Can you work these out from the model? Positions are in its coordinate system, mm. Give positions to 0.01 mm unless a question says otherwise; leave off trailing zeros. Loops run counter-clockwise (first coordinate to the right, second up) from the corner with the lowest first, then second, coordinate; pieces in that order, holes last.
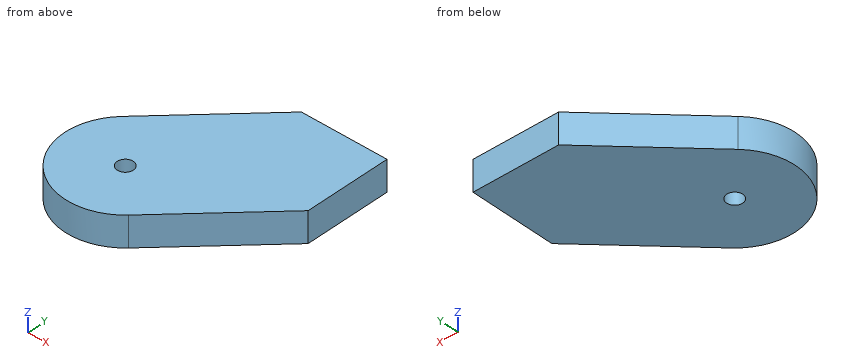
from build123d import *

# Parameters (mm, degrees)
F1_DEPTH = 25.4
F3_D     = 13.49248


with BuildPart() as f1:
    # F0 (on Top) → F1 (new body)
    with BuildSketch(Plane.XY):
        with BuildLine():
            Line((42.4579510314, 114.3), (-35.9210244843, 35.9210244843))
            ThreePointArc((-35.9210244843, 35.9210244843), (-35.9210244843, -35.9210244843), (35.9210244843, -35.9210244843))
            Line((35.9210244843, -35.9210244843), (114.3, 42.4579510314))
            Line((114.3, 42.4579510314), (114.3, 114.3))
            Line((114.3, 114.3), (42.4579510314, 114.3))
        make_face()
    extrude(amount=F1_DEPTH)

    # F3 (through all)
    with Locations(Plane.XY.offset(25.4)):
        with Locations((0, 0)):
            Hole(F3_D / 2)


solid = f1.part
(1) Suppose I cut it at D-D on x = 65.5. List the corners of the cut face in (y, z) for me, plus the area to 3 significant figures.
Returned:
outline: (-6.34, 0) - (114.3, 0) - (114.3, 25.4) - (-6.34, 25.4) - close
area: 3,060 mm2
(2) Please list where these lines run through material, in increasing order: probe 1 along Y at (x, z) = (0, 18.5); probe 2 along Y at (x, z) = (0.5, 18); probe 3 along Y at (x, z) = (70.5, 5.5).
Returned:
probe 1: y = -50.8 to -6.75, 6.75 to 71.84
probe 2: y = -50.8 to -6.73, 6.73 to 72.34
probe 3: y = -1.34 to 114.3
(3) Suppose I cut it at A-A on x = -1.5. List the corners of the cut face in (y, z) for me.
Returned:
outline: (-50.78, 0) - (-6.58, 0) - (-6.58, 25.4) - (-50.78, 25.4) - close; (6.58, 0) - (70.34, 0) - (70.34, 25.4) - (6.58, 25.4) - close
(4) Suppose I cut it at C-C on y = 0. List the corners of the cut face in (x, z) for me.
Returned:
outline: (-50.8, 0) - (-6.75, 0) - (-6.75, 25.4) - (-50.8, 25.4) - close; (6.75, 0) - (71.84, 0) - (71.84, 25.4) - (6.75, 25.4) - close
(5) Will these pins go through, and if not, where does the flat tip stop? P1, Ø1.5, axis at x = 40, z = 17, coming from the +Y side; P2, Ø10, axis at y = 36, z = 5, coming from the -X side; P3, Ø5, axis at x = 12, z = 18.5, coming from the -Y side.
Returned:
P1: stops at y = 112.59
P2: stops at x = -40.24
P3: stops at y = -49.9
(6) Suppose I cut it at B-B on z = 2.75. List the corners of the cut face in (x, y) for me.
Returned:
outline: (-35.92, 35.92) arc R50.8 ccw to (35.92, -35.92) - (114.3, 42.46) - (114.3, 114.3) - (42.46, 114.3) - close; hole circle Ø13.49 at (0, 0)
